```python
from build123d import *

# Parameters (mm, degrees)
SKETCH_1_R          = 3.25
SKETCH_1_R_2        = 2.25
SKETCH_1_R_3        = 1.75
EXTRUDE_1_DEPTH     = 0.3
SKETCH_1_4_R        = 2.25
SKETCH_1_4_R_2      = 1.75
EXTRUDE_2_DEPTH     = 5.5
CUT_EXTRUDE_1_DEPTH = 3.7
FILLET_1_R          = 0.05


with BuildPart() as part:
    # Sketch 1 → Extrude 1 (new body)
    with BuildSketch(Plane.XY):
        Circle(SKETCH_1_R)
        Circle(SKETCH_1_R_2, mode=Mode.SUBTRACT)
        Circle(SKETCH_1_R_2)
        Circle(SKETCH_1_R_3, mode=Mode.SUBTRACT)
    extrude(amount=EXTRUDE_1_DEPTH)

    # Sketch 1_4 → Extrude 2 (add)
    with BuildSketch(Plane.XY):
        Circle(SKETCH_1_4_R)
        Circle(SKETCH_1_4_R_2, mode=Mode.SUBTRACT)
    extrude(amount=-EXTRUDE_2_DEPTH)

    # Sketch 2 → Cut-Extrude 1 (cut)
    with BuildSketch(Plane(origin=(0, 0, -5.5), x_dir=(-1, 0, 0), z_dir=(0, 0, -1))):
        with BuildLine():
            ThreePointArc((-0.65, 2.154065923), (-2.25, 0), (-0.65, -2.154065923))
            Line((-0.65, -2.154065923), (-0.65, -1.624807681))
            ThreePointArc((-0.65, -1.624807681), (-1.75, 0), (-0.65, 1.624807681))
            Line((-0.65, 1.624807681), (-0.65, 2.154065923))
        make_face()
        with BuildLine():
            Line((0.65, -1.624807681), (0.65, -2.154065923))
            ThreePointArc((0.65, -2.154065923), (1.806239187, -1.341640786), (2.25, 0))
            ThreePointArc((2.25, 0), (1.806239187, 1.341640786), (0.65, 2.154065923))
            Line((0.65, 2.154065923), (0.65, 1.624807681))
            ThreePointArc((0.65, 1.624807681), (1.449137675, 0.981070844), (1.75, 0))
            ThreePointArc((1.75, 0), (1.449137675, -0.981070844), (0.65, -1.624807681))
        make_face()
    extrude(amount=-CUT_EXTRUDE_1_DEPTH, mode=Mode.SUBTRACT)

    # Fillet 1
    fillet_1_edges = [part.edges().sort_by_distance(p)[0] for p in [
        (0, 1.75, -5.5),
        (1.806239187, 1.341640786, -1.8),
        (0.65, -1.889436802, -5.5),
        (0.65, 1.889436802, -5.5),
        (0, -2.25, -5.5),
        (0, -1.75, -5.5),
        (-0.65, -1.889436802, -5.5),
        (-0.65, 1.889436802, -5.5),
        (-2.25, 0, -1.8),
        (-3.25, 0, 0),
        (-3.25, 0, 0.3),
        (0, 2.25, -5.5),
    ]]
    fillet(fillet_1_edges, radius=FILLET_1_R)


solid = part.part
```
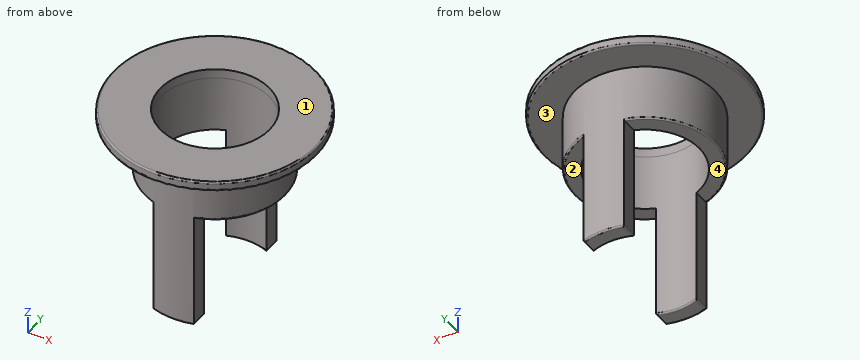
Build history of the part. All positions in model axes, mm. Face numbers are marked on the shaded views. A direction names the side the tool comes from. Coordinates: 2 decimals unless noted, no trailing zeros. Write each loop counter-clockwise with the first axis right and the second up, starting at its lowest first coordinate (ties: lowest second). Pieces come first, ordered by that corner, then holes.
1. Band-saw the part on B-B, the plane x = 0. Give the cut face in (y, z).
Answer block:
outline: (-3.25, 0.05) arc R0.05 ccw to (-3.2, 0) - (-2.25, 0) - (-2.25, -5.45) arc R0.05 ccw to (-2.2, -5.5) - (-1.8, -5.5) arc R0.05 ccw to (-1.75, -5.45) - (-1.75, 0.3) - (-3.2, 0.3) arc R0.05 ccw to (-3.25, 0.25) - close; (1.75, -5.45) arc R0.05 ccw to (1.8, -5.5) - (2.2, -5.5) arc R0.05 ccw to (2.25, -5.45) - (2.25, 0) - (3.2, 0) arc R0.05 ccw to (3.25, 0.05) - (3.25, 0.25) arc R0.05 ccw to (3.2, 0.3) - (1.75, 0.3) - close
2. Drill centre lines: probe 1 along Y at (x, z) = (0, 0.1); probe 2 along Y at (x, z) = (0, -2.3); probe 3 along Z at (x, y) = (-1, 1.75). Where is each one in solid material? Low to high.
Answer block:
probe 1: y = -3.25 to -1.75, 1.75 to 3.25
probe 2: y = -2.25 to -1.75, 1.75 to 2.25
probe 3: z = -1.8 to 0.3
3. Drop flat-ended pins along their axis: pin 1 (3 mm diameter, centred on x = 0, y = 0, fed in from +Z); pin 2 (0.8 mm diameter, centred on x = 1.5, y = 0, fed in from -Z); pin 3 (3 mm diameter, centred on y = 0.5, z = -4.5, fed in from +X); pin 4 (3 mm diameter, centred on x = -2, z = -2.5, fed in from -Y). Give the stop position or say it passes through.
Answer block:
pin 1: passes through
pin 2: stops at z = -1.8
pin 3: stops at x = 0.65
pin 4: stops at y = -2.19
4. 3-axis set-ups, long thin cutter, end or side, ignore diameter. For the marked faces 1, 2, 3 and 4: which of +Z, -Z, +X, -X, +Y, -Y reach the whole face in a straight line?
Answer block:
face 1: +Z, +X, -X, +Y, -Y
face 2: -Z, +X, +Y, -Y
face 3: -Z
face 4: -Z, -X, +Y, -Y
5. Band-saw the part on A-A, the plane z = -4.95. Give the cut face in (x, y).
Answer block:
outline: (-0.65, -2.15) arc R2.25 ccw to (0.65, -2.15) - (0.65, -1.62) arc R1.75 cw to (-0.65, -1.62) - close; (-0.65, 1.62) arc R1.75 cw to (0.65, 1.62) - (0.65, 2.15) arc R2.25 ccw to (-0.65, 2.15) - close
